Verification items for the finished model (mm, model axes). Face numbers are marked on the shaded views. A direction names the side the tool comes from. Round coordinates to 2 decimals unless told otherwise and drop trailing zeros. Write each loop counter-clockwise with the first axis right and the second up, starting at its lowest first coordinate (ties: lowest second). Pieces come first, ordered by that corner, then holes. Notation, with made-up numbers: M 22,86.5 L 80,86.5 A21 ccw 80,122.5 Z; hole C 86.5,80 d1. An arc over 180 degrees is marked long. Answer in a Markdown table with one row per item. Add a question column.
1. Draft check along Y on the marked faces 3, 4, 5 and 6. Enter one of: pulls with the +Y half, pulls with the -Y half, needs draft (parallel to the pull), parting line crosses it, or undercut.
2. Go/stop test with flat-tipped pins: pin 1 Ø1 at (x, y) = (33.5, -0.5) entering from +Z; pin 2 Ø1.8 at (x, y) = (30, -16.5) entering from -Z. Record where each tip stops, or that it passes through.
3. Sectioned sample at D-D on y = -31.5. Record the cut outline in (x, z).
4. Material ranges on probe 1 along Y at (x, z) = (29.5, 7.25); probe 2 along Y at (x, z) = (25.75, -9.25); probe 3 along Y at (x, z) = (26.5, -2.25), recorded low to high.
5. Set-up check for the marked faces 1 and 2: record each of +Z, -Z, +X, -X, +Y, -Y from which the full face is reachable in a straight line by a thin tool's end or side.
6. Sectioned sample at B-B on z = 6.5. Record the cut outline in (x, y).
7. Sectioned sample at C-C on x = 29.72. Record the cut outline in (y, z).
8. Sectioned sample at A-A on x = 25.91. Record the cut outline in (y, z).
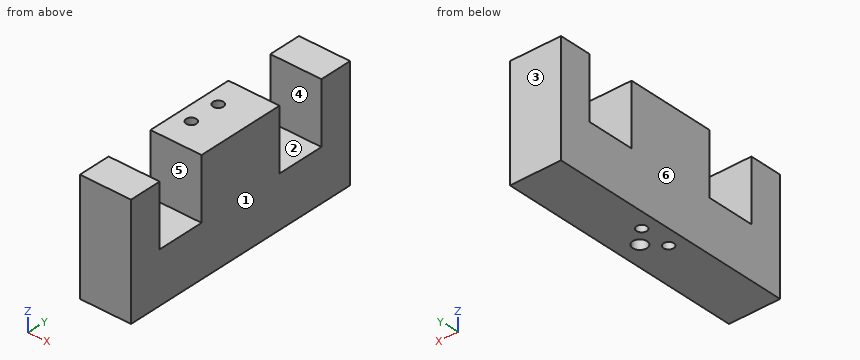
```python
from build123d import *

# Parameters (mm, degrees)
BOSS_EXTRUDE1_START = -4
SKETCH2_W           = 12.7
SKETCH2_H           = 11.829112303
SKETCH2_H_2         = 8.085443848
BOSS_EXTRUDE1_DEPTH = 12.7
BOSS_EXTRUDE3_START = -4
SKETCH2_4_W         = 12.7
SKETCH2_4_H         = 8.085443848
BOSS_EXTRUDE3_DEPTH = 15.24
SKETCH3_R           = 1.778
CUT_EXTRUDE1_DEPTH  = 7.62
SKETCH3_3_R         = 1.27
CUT_EXTRUDE2_DEPTH  = 66.423141131


with BuildPart() as part:
    # Sketch2 → Boss-Extrude1 (new body)
    with BuildSketch(Plane.XY.offset(BOSS_EXTRUDE1_START)):
        with BuildLine():
            Line((34.8, 12), (34.8, 14))
            Line((34.8, 14), (22.1, 14))
            Line((22.1, 14), (22.1, 5.914556152))
            Line((22.1, 5.914556152), (32.8, 5.914556152))
            ThreePointArc((32.8, 5.914556152), (34.214213562, 6.500342589), (34.8, 7.914556152))
            Line((34.8, 7.914556152), (34.8, 12))
        make_face()
        Polygon((32.8, 5.914556152), (22.1, 5.914556152), (22.1, -5.914556152), (32.8, -5.914556152), (34.8, -5.914556152), (34.8, 5.914556152), align=None)
        with BuildLine():
            Line((32.8, -5.914556152), (22.1, -5.914556152))
            Line((22.1, -5.914556152), (22.1, -27.923752717))
            Line((22.1, -27.923752717), (34.8, -27.923752717))
            Line((34.8, -27.923752717), (34.8, -12))
            Line((34.8, -12), (34.8, -7.914556152))
            ThreePointArc((34.8, -7.914556152), (34.214213562, -6.500342589), (32.8, -5.914556152))
        make_face()
        with Locations((28.45, -33.838308869)):
            Rectangle(SKETCH2_W, SKETCH2_H)
        with Locations((28.45, -43.795586944)):
            Rectangle(SKETCH2_W, SKETCH2_H_2)
        with BuildLine():
            Line((34.8, 5.914556152), (34.8, 7.914556152))
            ThreePointArc((34.8, 7.914556152), (34.214213562, 6.500342589), (32.8, 5.914556152))
            Line((32.8, 5.914556152), (34.8, 5.914556152))
        make_face()
        with BuildLine():
            Line((34.8, -5.914556152), (32.8, -5.914556152))
            ThreePointArc((32.8, -5.914556152), (34.214213562, -6.500342589), (34.8, -7.914556152))
            Line((34.8, -7.914556152), (34.8, -5.914556152))
        make_face()
    extrude(amount=-BOSS_EXTRUDE1_DEPTH)

    # Sketch2<4> → Boss-Extrude3 (add)
    with BuildSketch(Plane.XY.offset(BOSS_EXTRUDE3_START)):
        with BuildLine():
            Line((34.8, 12), (34.8, 14))
            Line((34.8, 14), (22.1, 14))
            Line((22.1, 14), (22.1, 5.914556152))
            Line((22.1, 5.914556152), (32.8, 5.914556152))
            ThreePointArc((32.8, 5.914556152), (34.214213562, 6.500342589), (34.8, 7.914556152))
            Line((34.8, 7.914556152), (34.8, 12))
        make_face()
        with BuildLine():
            Line((34.8, 5.914556152), (34.8, 7.914556152))
            ThreePointArc((34.8, 7.914556152), (34.214213562, 6.500342589), (32.8, 5.914556152))
            Line((32.8, 5.914556152), (34.8, 5.914556152))
        make_face()
        with BuildLine():
            Line((32.8, -5.914556152), (22.1, -5.914556152))
            Line((22.1, -5.914556152), (22.1, -27.923752717))
            Line((22.1, -27.923752717), (34.8, -27.923752717))
            Line((34.8, -27.923752717), (34.8, -12))
            Line((34.8, -12), (34.8, -7.914556152))
            ThreePointArc((34.8, -7.914556152), (34.214213562, -6.500342589), (32.8, -5.914556152))
        make_face()
        with BuildLine():
            Line((34.8, -5.914556152), (32.8, -5.914556152))
            ThreePointArc((32.8, -5.914556152), (34.214213562, -6.500342589), (34.8, -7.914556152))
            Line((34.8, -7.914556152), (34.8, -5.914556152))
        make_face()
        with Locations((28.45, -43.795586944)):
            Rectangle(SKETCH2_4_W, SKETCH2_4_H)
    extrude(amount=BOSS_EXTRUDE3_DEPTH)

    # Sketch3 → Cut-Extrude1 (cut)
    with BuildSketch(Plane(origin=(0, 0, -16.7), x_dir=(-1, 0, 0), z_dir=(0, 0, -1))):
        with Locations((-29.72, -16.919154434)):
            Circle(SKETCH3_R)
    extrude(amount=-CUT_EXTRUDE1_DEPTH, mode=Mode.SUBTRACT)

    # Sketch3<3> → Cut-Extrude2 (cut, through all)
    with BuildSketch(Plane(origin=(0, 0, -16.7), x_dir=(-1, 0, 0), z_dir=(0, 0, -1))):
        with Locations((-25.91, -13.109154434)):
            Circle(SKETCH3_3_R)
        with Locations((-25.91, -20.729154434)):
            Circle(SKETCH3_3_R)
    extrude(amount=-CUT_EXTRUDE2_DEPTH, mode=Mode.SUBTRACT)


solid = part.part
```
Geometry check:
| question | item | result |
|---|---|---|
| 1 | face 3 | pulls with the +Y half |
| 1 | face 4 | undercut |
| 1 | face 5 | undercut |
| 1 | face 6 | needs draft |
| 2 | pin 1 | stops at z = -4 |
| 2 | pin 2 | stops at z = -9.08 |
| 3 | outline | M 22.1,-16.7 L 34.8,-16.7 L 34.8,-4 L 22.1,-4 Z |
| 4 | probe 1 | y = -47.84 to -39.75, -27.92 to -5.91, 5.91 to 14 |
| 4 | probe 2 | y = -47.84 to -21.99, -19.47 to -14.37, -11.85 to 14 |
| 4 | probe 3 | y = -47.84 to -39.75, -27.92 to -21.85, -19.6 to -14.23, -11.98 to -5.91, 5.91 to 14 |
| 5 | face 1 | +Z, -Z, +X, +Y, -Y |
| 5 | face 2 | +Z, +X, -X |
| 6 | outline | M 22.1,-47.84 L 34.8,-47.84 L 34.8,-39.75 L 22.1,-39.75 Z; M 22.1,-27.92 L 34.8,-27.92 L 34.8,-5.91 L 22.1,-5.91 Z; M 22.1,5.91 L 34.8,5.91 L 34.8,14 L 22.1,14 Z; hole C 25.91,-20.73 d2.54; hole C 25.91,-13.11 d2.54 |
| 7 | outline | M -47.84,-16.7 L -18.7,-16.7 L -18.7,-9.08 L -15.14,-9.08 L -15.14,-16.7 L 14,-16.7 L 14,11.24 L 5.91,11.24 L 5.91,-4 L -5.91,-4 L -5.91,11.24 L -27.92,11.24 L -27.92,-4 L -39.75,-4 L -39.75,11.24 L -47.84,11.24 Z |
| 8 | outline | M -47.84,-16.7 L -22,-16.7 L -22,11.24 L -27.92,11.24 L -27.92,-4 L -39.75,-4 L -39.75,11.24 L -47.84,11.24 Z; M -19.46,-16.7 L -14.38,-16.7 L -14.38,11.24 L -19.46,11.24 Z; M -11.84,-16.7 L 14,-16.7 L 14,11.24 L 5.91,11.24 L 5.91,-4 L -5.91,-4 L -5.91,11.24 L -11.84,11.24 Z |
